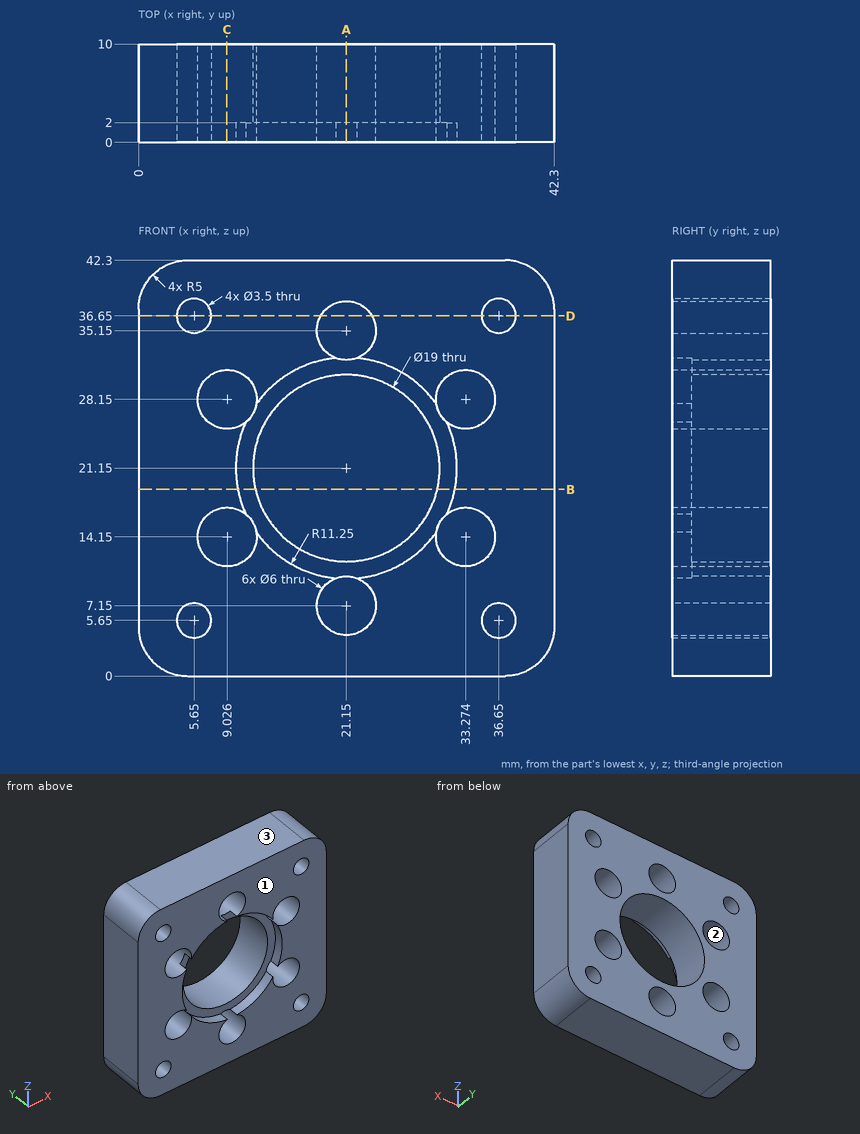
Design review of the part shown in the three views and the two pictorial views. Dimensions are in mm from the part's minimum x, y and z. Give positions to 0.01 mm unless a question says otherwise; leave off trailing zeros. Write each loop counter-clockwise with the first axis right and the second up, starting at its lowest first coordinate (ties: lowest second). Pieces come first, ordered by that corner, then holes. Notation, with made-up numbers: M 47.5,51.5 L 62.5,51.5 A22 cw 62.5,58.5 Z; hole C 37,38 d2. An arc over 180 degrees is marked long. One line per item, written item: value.
1) Take a section at D-D, the plane z = 36.65. Write out the cut boundary in (x, y), then the cut area to 3 significant figures.
Results are:
outline: M 0,0 L 3.9,0 L 3.9,10 L 0,10 Z; M 7.4,0 L 18.55,0 L 18.55,10 L 7.4,10 Z; M 23.75,0 L 34.9,0 L 34.9,10 L 23.75,10 Z; M 38.4,0 L 42.3,0 L 42.3,10 L 38.4,10 Z
area: 301 mm²
2) Take a section at C-C, the plane x = 9. Write out the cut boundary in (y, z), then the cut area to 3 significant figures.
Results are:
outline: M 0,0 L 10,0 L 10,11.15 L 0,11.15 Z; M 0,17.15 L 10,17.15 L 10,25.15 L 0,25.15 Z; M 0,31.15 L 10,31.15 L 10,42.3 L 0,42.3 Z
area: 303 mm²
3) Take a section at B-B, the plane z = 19. Write out the cut boundary in (x, y), then the cut area to 3 significant figures.
Results are:
outline: M 0,0 L 10.11,0 L 10.11,2 L 11.9,2 L 11.9,10 L 0,10 Z; M 30.4,2 L 32.19,2 L 32.19,0 L 42.3,0 L 42.3,10 L 30.4,10 Z
area: 231 mm²
4) Take a section at A-A, the plane x = 21.15. Write out the cut boundary in (y, z), then the cut area to 3 significant figures.
Results are:
outline: M 0,0 L 10,0 L 10,4.15 L 0,4.15 Z; M 0,38.15 L 10,38.15 L 10,42.3 L 0,42.3 Z; M 2,10.15 L 10,10.15 L 10,11.65 L 2,11.65 Z; M 2,30.65 L 10,30.65 L 10,32.15 L 2,32.15 Z
area: 107 mm²
5) For line 1 (Z direction, x = 36.5, y = 5.5); line 2 (X direction, y = 2.25, z = 37) (1 decimal); line 3 (X direction, y = 7.75, z = 14.15) (1 decimal), list the stretches that pass through material, from the lowest coordinate up. Write a range as from..to.
Results are:
line 1: z = 0..3.91, 7.39..34.91, 38.39..42.3
line 2: x = 0..3.9, 7.4..18.8, 23.5..34.9, 38.4..42.3
line 3: x = 0..6, 12..14.7, 27.6..30.3, 36.3..42.3
6) The part is to be moulded in two halves that separate along Z. For the marked faces 1, 2 and 3, say which applies: +Z half, -Z half, draft (parallel to the pull), parting line (faces both ways), or undercut.
Results are:
face 1: draft
face 2: undercut
face 3: +Z half
